from build123d import *

# Parameters (mm, degrees)
F2_R     = 7.5
F3_DEPTH = 33


with BuildPart() as f1:
    # F0 (on Right) → F1 (revolve)
    with BuildSketch(Plane.YZ):
        with BuildLine():
            Line((-12.0403646417, 39), (-12.0403646417, 31))
            Line((-12.0403646417, 31), (23.4514921904, 29))
            Line((23.4514921904, 29), (23.4514921904, 26))
            Line((23.4514921904, 26), (65.4514921904, 26))
            Line((65.4514921904, 26), (65.4514921904, 0))
            Line((65.4514921904, 0), (77.9596353583, 0))
            Line((77.9596353583, 0), (77.9596353583, 32))
            Line((77.9596353583, 32), (80.9596353583, 32))
            Line((80.9596353583, 32), (80.9596353583, 39))
            Line((80.9596353583, 39), (47.9596353583, 39))
            Line((47.9596353583, 39), (33.8275175401, 29.1045845728))
            ThreePointArc((33.8275175401, 29.1045845728), (28.6508922921, 28.7652906284), (25.9596353583, 33.2003447942))
            Line((25.9596353583, 33.2003447942), (25.9596353583, 39))
            Line((25.9596353583, 39), (25.9596353583, 45))
            Line((25.9596353583, 45), (-4.0403646417, 45))
            Line((-4.0403646417, 45), (-4.0403646417, 39))
            Line((-4.0403646417, 39), (-12.0403646417, 39))
        make_face()
    revolve(axis=Axis((0, 71.7055637743, 0), (0, -1, 0)))

    # F2 (on face) → F3 (join)
    with BuildSketch(Plane(origin=(0, 80.9596353583, 0), x_dir=(-1, 0, 0), z_dir=(0, 1, 0))):
        with BuildLine():
            Line((36.6079755837, 13.4482758621), (17.8346547716, 64.5517241379))
            ThreePointArc((17.8346547716, 64.5517241379), (0, 77), (-17.8346547716, 64.5517241379))
            Line((-17.8346547716, 64.5517241379), (-36.6079755837, 13.4482758621))
            ThreePointArc((-36.6079755837, 13.4482758621), (0, 39), (36.6079755837, 13.4482758621))
        make_face()
        with Locations((0, 58)):
            Circle(F2_R, mode=Mode.SUBTRACT)
        with BuildLine():
            Line((17.8346547716, -64.5517241379), (36.6079755837, -13.4482758621))
            ThreePointArc((36.6079755837, -13.4482758621), (0, -39), (-36.6079755837, -13.4482758621))
            Line((-36.6079755837, -13.4482758621), (-17.8346547716, -64.5517241379))
            ThreePointArc((-17.8346547716, -64.5517241379), (0, -77), (17.8346547716, -64.5517241379))
        make_face()
        with Locations((0, -58)):
            Circle(F2_R, mode=Mode.SUBTRACT)
    extrude(amount=-F3_DEPTH)


solid = f1.part
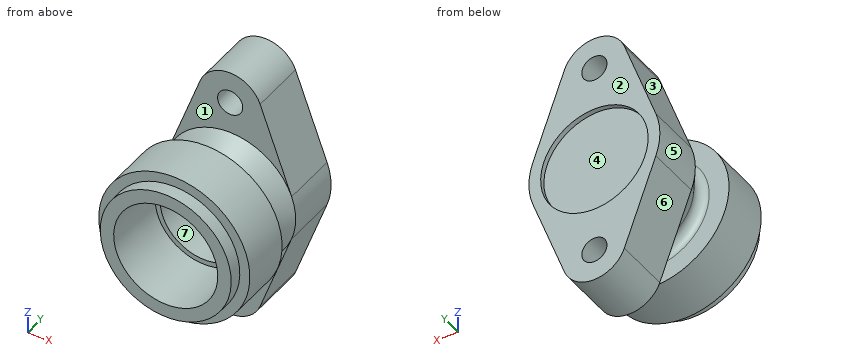
Could you check a few things on this model? Use its own coordinates, in mm. Face numbers are marked on the shaded views. A direction names the side the tool comes from. Give positions to 0.01 mm unless a question says otherwise; leave off trailing zeros. Order: outer loops, then holes, each group sorted by start corner. A loop starts at its lowest first (then second) coordinate and runs counter-clockwise, first axis right, second up. Notation, with made-up numbers: M 63.5,9 L 92.5,9 A21 cw 92.5,17 Z; hole C 50.25,28.5 d9. An arc over 180 degrees is marked long. One line per question, with ' | ' between items.
1. I'm going to push flat-ended pins straight in: pin 1 (6 mm diameter, centred on x = 29.5, z = -46, fed in from -Y); pin 2 (5 mm diameter, centred on y = 60, z = 34, fed in from +X); pin 3 (12 mm diameter, centred on x = -4.5, y = 12, fed in from -Z); pin 4 (12 mm diameter, centred on x = 20, y = 56, fed in from -Z). Where does each tip first touch, or does it pass through?
Results:
pin 1: through | pin 2: x = 29.98 | pin 3: z = -45 | pin 4: z = -70.85
2. I want a section at B-B (z = 58). List the corners of the cut face in (x, y) for me.
Results:
outline: M -20.24,47.96 L -7.5,47.96 L -7.5,80.96 L -20.24,80.96 Z; M 7.5,47.96 L 20.24,47.96 L 20.24,80.96 L 7.5,80.96 Z
3. If I drill on line 1 (Y direction, x = 20.5, z = 34.5); line 2 (Y direction, x = 6.5, z = -64); line 3 (Y direction, x = 6, z = 4.5), over which ranges is the centre line in solid material (lowest first)?
Results:
line 1: -4.04 to 25.96, 47.96 to 80.96 | line 2: 47.96 to 80.96 | line 3: 65.45 to 77.96
4. I want a section at C-C (z = 0). List the corners of the cut face in (x, y) for me, and give its area (3 significant figures).
Results:
outline: M -45,-4.04 L -39,-4.04 L -39,-12.04 L -31,-12.04 L -29,23.45 L -26,23.45 L -26,65.45 L 26,65.45 L 26,23.45 L 29,23.45 L 31,-12.04 L 39,-12.04 L 39,-4.04 L 45,-4.04 L 45,25.96 L 33.2,25.96 A5 cw 29.1,33.83 L 39,47.96 L 39,80.96 L 32,80.96 L 32,77.96 L -32,77.96 L -32,80.96 L -39,80.96 L -39,47.96 L -29.1,33.83 A5 cw -33.2,25.96 L -45,25.96 Z | area: 2,810 mm²
5. For the marked faces 4, 5, 6 and 7, which set-ups out of +Z, -Z, +X, -X, +Y, -Y let a thin tool reach every point of the face, with its end or its side?
Results:
face 4: +Y | face 5: -X, +Y | face 6: -Z, -X, +Y | face 7: -Y
6. We'd pull the mould along Y, two halves only. Please class the marked faces 1, 2 and 3: +Y half, -Y half, draft (parallel to the pull), parting line (faces both ways), or undercut.
Results:
face 1: undercut | face 2: +Y half | face 3: draft
7. I want a section at A-A (y = 52.5). List the corners of the cut face in (x, z) for me.
Results:
outline: M -36.61,-13.45 L -17.83,-64.55 A19 ccw 17.83,-64.55 L 36.61,-13.45 A39 ccw 36.61,13.45 L 17.83,64.55 A19 ccw -17.83,64.55 L -36.61,13.45 A39 ccw Z; hole C 0,0 d52; hole C 0,-58 d15; hole C 0,58 d15
8. I want a section at D-D (y = 18). List the corners of the cut face in (x, z) for me.
Results:
outline: C 0,0 d90; hole C 0,0 d58.61
